Here's how the part is built. I have some questions about the finished solid (model axes, mm). A direction names the side the tool comes from. Round coordinates to 2 decimals unless told otherwise and drop trailing zeros. Loops run counter-clockwise (first coordinate to the right, second up) from the corner with the lowest first, then second, coordinate; pieces in that order, holes last. Notation, with made-up numbers: M -12,-21 L 24,-21 A30 cw 24,1 Z; hole C -21.5,78.25 d1. An arc over 180 degrees is marked long. Use a Markdown table: item, result.
```python
from build123d import *

# Parameters (mm, degrees)
F0_R     = 10.5
F1_DEPTH = 3
F2_SIZE  = 1
F3_R     = 9.5
F4_DEPTH = 3


with BuildPart() as f1:
    # F0 (on Top) → F1 (new body)
    with BuildSketch(Plane.XY):
        Circle(F0_R)
    extrude(amount=F1_DEPTH)

    # F2
    f2_edges = [f1.edges().sort_by_distance(p)[0] for p in [
        (-10.5, 0, 0),
    ]]
    chamfer(f2_edges, length=F2_SIZE)

    # F3 (on face) → F4 (join)
    with BuildSketch(Plane.XY.offset(3)):
        Circle(F3_R)
    extrude(amount=F4_DEPTH)


solid = f1.part
```
Q1. Imagine slicing it at C-C, the plane z = 4.65. Please give me the cut outline in (x, y).
Return value:
| item | result |
|---|---|
| outline | C 0,0 d19 |
Q2. I need wall thicknesses on line 1 (X direction, y = 8, z = 0.75); line 2 (Y direction, x = 7.5, z = 2.5); line 3 (X direction, y = 5.25, z = 5.45). Which ranges of each line are inside material? Lowest first, please. Write a range as from..to.
Return value:
| item | result |
|---|---|
| line 1 | x = -6.41..6.41 |
| line 2 | y = -7.35..7.35 |
| line 3 | x = -7.92..7.92 |
Q3. For faces 1 (the flat face through (0, 0, 0)), 2 (the cylindrical face through (4.38, -8.43, 4.48)), which set-ups out of +Z, -Z, +X, -X, +Y, -Y let a thin tool reach every point of the face, with its end or its side?
Return value:
| item | result |
|---|---|
| face 1 | -Z, +X, -X, +Y, -Y |
| face 2 | +Z |
Q4. Imagine slicing it at D-D, the plane z = 0.75. Please give me the cut outline in (x, y).
Return value:
| item | result |
|---|---|
| outline | C 0,0 d20.5 |
Q5. Imagine slicing it at A-A, the plane y = 0. Please give me the cut outline in (x, z).
Return value:
| item | result |
|---|---|
| outline | M -10.5,1 L -9.5,0 L 9.5,0 L 10.5,1 L 10.5,3 L 9.5,3 L 9.5,6 L -9.5,6 L -9.5,3 L -10.5,3 Z |
Q6. Will this pin go through, and if not, where does the flat tip stop? P1, Ø12, axis at x = 7, y = 7.5, coming from the -Z side.
Return value:
| item | result |
|---|---|
| P1 | stops at z = 0 |
